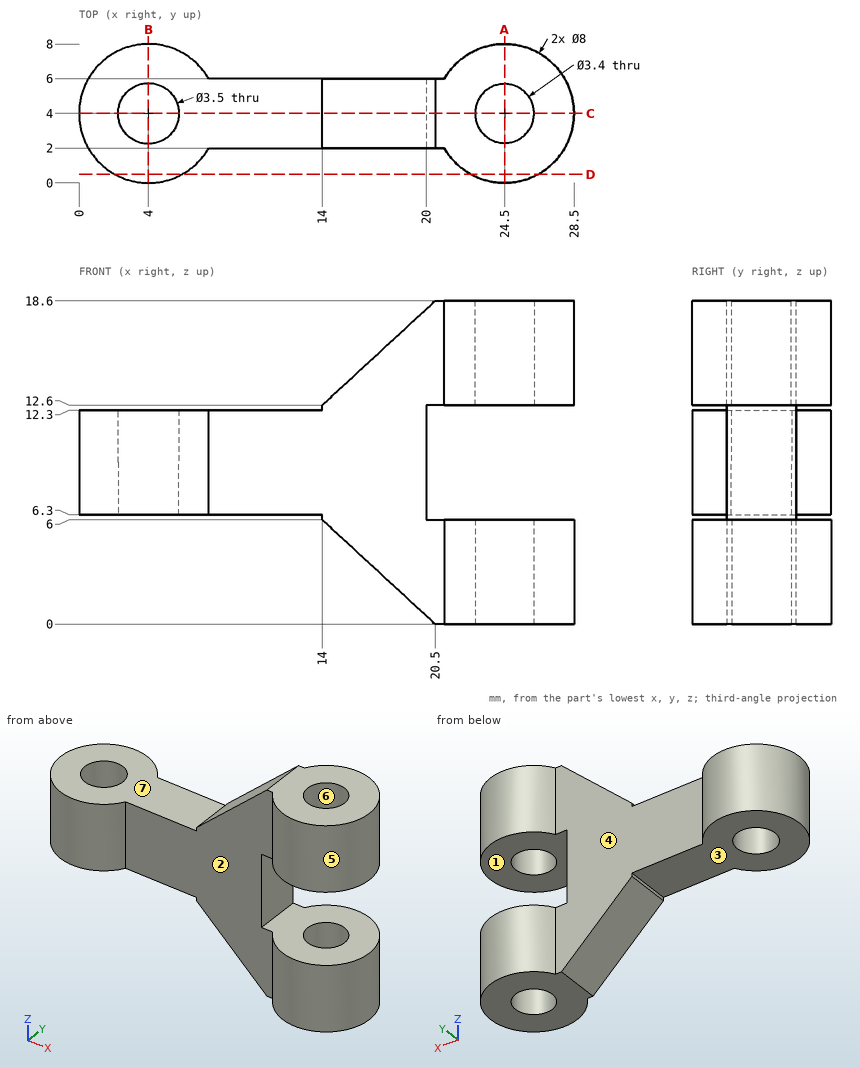
Source: three-view drawing plus pictorial views. Frame: mm from the lowest corner of the part. A direction names the side the tool comes from. Round coordinates to 2 decimals unless told otherwise and drop trailing zeros. Loops run counter-clockwise (first coordinate to the right, second up) from the corner with the lowest first, then second, coordinate; pieces in that order, holes last. Notation, with made-up numbers: (-15, 44) - (19, 44) arc R20 cw to (19, 80) - close; hole circle Ø7 at (17.25, -7.75). An arc over 180 degrees is marked (long way). Write item = value, one per line. Start each with the question number.
Item 1: Section query C-C on y = 4. Output: boundary loops of the cut face in (x, z), plus the area to 3 significant figures.
Item 2: First-contact query: pin 1 Ø11 at (x, z) = (16.5, 5) entering from -Y; pin 2 Ø3 at (y, z) = (4, 9) entering from +X; pin 3 Ø4 at (x, y) = (9.5, 3) entering from +Z. Flat tips, straight axial feed; report the tip coordinate or a pass-through.
Item 3: Section query A-A on x = 24.5. Output: boundary loops of the cut face in (y, z).
Item 4: Reachability of the marked faces 1, 2, 3 and 4 from +Z, -Z, +X, -X, +Y, -Y: full face, straight path, thin tool, end or side. Return the list, or none.
Item 5: Section query B-B on x = 4. Output: boundary loops of the cut face in (y, z), plus the area to 3 significant figures.
Item 6: Mould query, pull axis X, two halves, no side actions, for the marked faces 5, 6 and 7. Classes: released by +X, released by -X, zero draft, split by the parting line, or undercut.
Item 7: Material intervals for line 1 (Y direction, x = 24.5, z = 15.7); line 2 (Y direction, x = 23.5, z = 3.5); line 3 (X direction, y = 4.25, z = 1.25), sorted ascending.
Item 8: Section query D-D on y = 0.5. Output: boundary loops of the cut face in (x, z).
Results list:
q1.outline = (0, 6.3) - (2.25, 6.3) - (2.25, 12.3) - (0, 12.3) - close; (5.75, 6.3) - (14, 6.3) - (14, 6) - (20.5, 0) - (22.8, 0) - (22.8, 6) - (20, 6) - (20, 12.6) - (22.8, 12.6) - (22.8, 18.6) - (20.5, 18.6) - (14, 12.6) - (14, 12.3) - (5.75, 12.3) - close; (26.2, 0) - (28.5, 0) - (28.5, 6) - (26.2, 6) - close; (26.2, 12.6) - (28.5, 12.6) - (28.5, 18.6) - (26.2, 18.6) - close
q1.area = 197 mm²
q2.pin_1 = 0.88
q2.pin_2 = 20
q2.pin_3 = 12.3
q3.outline = (0, 0) - (2.3, 0) - (2.3, 6) - (0, 6) - close; (0, 12.6) - (2.3, 12.6) - (2.3, 18.6) - (0, 18.6) - close; (5.7, 0) - (8, 0) - (8, 6) - (5.7, 6) - close; (5.7, 12.6) - (8, 12.6) - (8, 18.6) - (5.7, 18.6) - close
q4.face_1 = +X, +Y, -Y
q4.face_2 = +Z, -Z, -Y
q4.face_3 = -Z, -X, +Y, -Y
q4.face_4 = +Z, -Z, +Y
q5.outline = (0, 6.3) - (2.25, 6.3) - (2.25, 12.3) - (0, 12.3) - close; (5.75, 6.3) - (8, 6.3) - (8, 12.3) - (5.75, 12.3) - close
q5.area = 27.0 mm²
q6.face_5 = split by the parting line
q6.face_6 = undercut
q6.face_7 = zero draft
q7.line_1 = 0 to 2.3, 5.7 to 8
q7.line_2 = 0.13 to 2.63, 5.37 to 7.87
q7.line_3 = 19.15 to 22.82, 26.18 to 28.49
q8.outline = (2.06, 6.3) - (5.94, 6.3) - (5.94, 12.3) - (2.06, 12.3) - close; (22.56, 0) - (26.44, 0) - (26.44, 6) - (22.56, 6) - close; (22.56, 12.6) - (26.44, 12.6) - (26.44, 18.6) - (22.56, 18.6) - close
